Geometry: final body of the model. Coordinates: model frame, mm. A direction names the side the tool comes from. Give positions to 0.01 mm unless a question says otherwise; leave off trailing zeros. Loops run counter-clockwise (first coordinate to the right, second up) from the corner with the lowest first, then second, coordinate; pieces in that order, holes last. Notation, with made-up numbers: M 36.5,47.25 L 53.5,47.25 A22 ccw 53.5,80.25 Z; hole C -16,-5.75 d1. An arc over 180 degrees is marked long. Put each result on its own line as item: value.
```python
from build123d import *

# Parameters (mm, degrees)
SKETCH1_R           = 7.75
BOSS_EXTRUDE1_DEPTH = 240
BOSS_EXTRUDE2_DEPTH = 10


with BuildPart() as part:
    # Sketch1 → Boss-Extrude1 (new body)
    with BuildSketch(Plane(origin=(0, 0, 0), x_dir=(0, 0, -1), z_dir=(1, 0, 0))):
        Circle(SKETCH1_R)
    boss_extrude1 = extrude(amount=BOSS_EXTRUDE1_DEPTH)

    # Sketch2 → Boss-Extrude2 (add)
    with BuildSketch(Plane(origin=(240, 0, 0), x_dir=(0, 0, -1), z_dir=(1, 0, 0))):
        with BuildLine():
            Line((-7.8, 0), (-7.8, -10.2))
            Line((-7.8, -10.2), (-11.9, -10.2))
            Line((-11.9, -10.2), (-11.9, -21.2))
            Line((-11.9, -21.2), (11.9, -21.2))
            Line((11.9, -21.2), (11.9, -10.2))
            Line((11.9, -10.2), (7.8, -10.2))
            Line((7.8, -10.2), (7.8, 0))
            ThreePointArc((7.8, 0), (0, 7.8), (-7.8, 0))
        make_face()
    boss_extrude2 = extrude(amount=BOSS_EXTRUDE2_DEPTH)

    # Mirror1: Boss-Extrude1, Boss-Extrude2 across plane
    add(boss_extrude1.mirror(Plane.ZY))
    add(boss_extrude2.mirror(Plane.ZY))


solid = part.part
```
Item 1: Line query: probe 1 along X at (y, z) = (-11.75, 7); probe 2 along Z at (x, y) = (142.5, -0.5); probe 3 along Y at (x, z) = (-11.5, -3.75). Output: solid intervals per line, ascending. Write a range as [from, to].
Output values:
probe 1: [-250, -240], [240, 250]
probe 2: [-7.73, 7.73]
probe 3: [-6.78, 6.78]
Item 2: Pin query (flat end, axial travel): pin 1 Ø2 at (x, z) = (244, -10.5) entering from +Y; pin 2 Ø11 at (x, y) = (-247.5, -3) entering from +Z; pin 3 Ø3 at (x, y) = (244, -4) entering from -Z. Return the tip coordinate at first contact, or that it passes through.
Output values:
pin 1: y = -10.2
pin 2: z = 7.8
pin 3: z = -7.8
Item 3: Section B-B on x = 82. Output: boundary loops of the cut face in (y, z), then the cut area to 3 significant figures.
Output values:
outline: C 0,0 d15.5
area: 189 mm²
Item 4: Section A-A on z = 0. Output: boundary loops of the cut face in (x, y).
Output values:
outline: M -250,-21.2 L -240,-21.2 L -240,-7.75 L 240,-7.75 L 240,-21.2 L 250,-21.2 L 250,7.8 L 240,7.8 L 240,7.75 L -240,7.75 L -240,7.8 L -250,7.8 Z
Item 5: Set-up query: faces 5 (the flat face through (245, -5, 7.8)), 6 (the cylindrical face through (-244.93, 7.8, -0.17)), 7 (the flat face through (-245, -5, -7.8)). Return all of +Z, -Z, +X, -X, +Y, -Y with unobstructed straight access to the full face (end or side cutting, diameter ignored); none if empty.
Output values:
face 5: +Z, +X, -X, +Y
face 6: +X, -X, +Y
face 7: -Z, +X, -X, +Y
Item 6: Mould query, pull axis X, two halves, no side actions, for faces 1 (the flat face through (-250, -10, 0)), 2 (the cylindrical face through (244.93, 7.8, -0.17)), 3 (the cylindrical face through (3.36, 7.684, 1.009)), 4 (the flat face through (240, -13, 0)). Classes: pulls with the +X half, pulls with the -X half, needs draft (parallel to the pull), parting line crosses it, or undercut.
Output values:
face 1: pulls with the -X half
face 2: needs draft
face 3: undercut
face 4: undercut
